```python
from build123d import *

# Parameters (mm, degrees)
F0_R     = 1.5
F0_R_2   = 11
F1_DEPTH = 40
F0_R_3   = 2.5
F2_DEPTH = 42
F3_DEPTH = 60
F4_DEPTH = 35


with BuildPart() as f1:
    # F0 (on Front) → F1 (new body)
    with BuildSketch(Plane.XZ):
        Polygon((-16.5, -21.15), (16.5, -21.15), (21.15, -16.5), (21.15, 16.5), (16.5, 21.15), (-16.5, 21.15), (-21.15, 16.5), (-21.15, -16.5), align=None)
        with Locations((-15.5, -15.5)):
            Circle(F0_R, mode=Mode.SUBTRACT)
        with Locations((15.5, -15.5)):
            Circle(F0_R, mode=Mode.SUBTRACT)
        with Locations((-15.5, 15.5)):
            Circle(F0_R, mode=Mode.SUBTRACT)
        Circle(F0_R_2, mode=Mode.SUBTRACT)
        with Locations((15.5, 15.5)):
            Circle(F0_R, mode=Mode.SUBTRACT)
    extrude(amount=F1_DEPTH)

    # F0 (on Front) → F2 (join)
    with BuildSketch(Plane.XZ):
        Circle(F0_R_2)
        Circle(F0_R_3, mode=Mode.SUBTRACT)
    extrude(amount=F2_DEPTH)

    # F0 (on Front) → F3 (join)
    with BuildSketch(Plane.XZ):
        Circle(F0_R_3)
    extrude(amount=F3_DEPTH)

    # F0 (on Front) → F4 (join)
    with BuildSketch(Plane.XZ):
        with Locations((15.5, 15.5)):
            Circle(F0_R)
        with Locations((-15.5, 15.5)):
            Circle(F0_R)
        with Locations((-15.5, -15.5)):
            Circle(F0_R)
        with Locations((15.5, -15.5)):
            Circle(F0_R)
    extrude(amount=F4_DEPTH)


solid = f1.part
```
The listing builds one solid part. Answer for the finished solid, in the listing's coordinates (mm). A direction names the side the tool comes from. Round coordinates to 2 decimals unless told otherwise and drop trailing zeros. Order: outer loops, then holes, each group sorted by start corner. A loop starts at its lowest first (then second) coordinate and runs counter-clockwise, first axis right, second up. Notation, with made-up numbers: (59.5, -9.5) - (98.5, -9.5) arc R18 cw to (98.5, 23.5) - close; hole circle Ø9 at (-4.75, 62.25). An arc over 180 degrees is marked (long way). Put each result on its own line as item: value. Start each with the question number.
(1) Given P1, Ø3.5, axis at x = -15.5, z = -16, coming from the -Y side; P2, Ø1.5, axis at x = 15.5, z = -15.5, coming from the -Y side; P3, Ø6, axis at x = 1, y = -48, coming from the +Z side, each flat-ended and moving along its own axis, determine where each tip first touches the part or whether it passes through.
(2) Find section B-B (x = 0). Give the vertices of the cut face in (y, z).
(3) Determine the mould class of faces 3 (the flat face through (15, -35, 16)), 4 (the flat face through (-18.79, -19.72, 18.86)), 5 (the flat face through (18.79, -19.72, -18.86)) for opening direction Z: released by +Z, released by -Z, zero draft, split by the parting line, or undercut.
(4) Find section D-D (z = -4). Give the vertices of the cut face in (x, y).
(5) Straight lines are drawn through the part: probe 1 along Z at (x, y) = (-15.5, -38.55); probe 2 along X at (y, z) = (-38, 15); probe 3 along Y at (x, z) = (-17, 14). For each, find the intervals that lie inside material, in ascending order. Write a range as from..to.
(6) Find section A-A (z = -15.5). Give the vertices of the cut face in (x, y), plus the area to 3 significant figures.
(7) Find section C-C (y = -19). Give the vertices of the cut face in (x, z), plus the area to 3 significant figures.
(8) For faces 1 (the flat face through (9, -40, -9)), 2 (the flat face through (18.86, -19.72, 18.79)), determine the directions among +Z, -Z, +X, -X, +Y, -Y from which every point of the face is accessible in a straight line to the end or side of a thin tool.
Reply:
1. P1: y = -40
1. P2: y = -35
1. P3: z = 2.5
2. outline: (-60, -2.5) - (-42, -2.5) - (-42, -11) - (-40, -11) - (-40, -21.15) - (0, -21.15) - (0, 21.15) - (-40, 21.15) - (-40, 11) - (-42, 11) - (-42, 2.5) - (-60, 2.5) - close
3. face 3: undercut
3. face 4: released by +Z
3. face 5: released by -Z
4. outline: (-21.15, -40) - (-10.25, -40) - (-10.25, -42) - (10.25, -42) - (10.25, -40) - (21.15, -40) - (21.15, 0) - (-21.15, 0) - close
5. probe 1: -21.15..-17, -14..14, 17..21.15
5. probe 2: -21.15..-16.91, -14.09..14.09, 16.91..21.15
5. probe 3: -40..0
6. outline: (-21.15, -40) - (-17, -40) - (-17, -35) - (-14, -35) - (-14, -40) - (14, -40) - (14, -35) - (17, -35) - (17, -40) - (21.15, -40) - (21.15, 0) - (-21.15, 0) - close
6. area: 1,660 mm^2
7. outline: (-21.15, -16.5) - (-16.5, -21.15) - (16.5, -21.15) - (21.15, -16.5) - (21.15, 16.5) - (16.5, 21.15) - (-16.5, 21.15) - (-21.15, 16.5) - close
7. area: 1,750 mm^2
8. face 1: -Y
8. face 2: +Z, +X, +Y, -Y
